from build123d import *

# Parameters (mm, degrees)
SKETCH1_W               = 53
SKETCH1_H               = 53
BOSS_EXTRUDE1_DEPTH     = 1.5
SKETCH2_W               = 16
SKETCH2_H               = 9
CUT_EXTRUDE1_DEPTH      = 75.968326645
SKETCH3_W               = 4.5
SKETCH3_H               = 8
BOSS_EXTRUDE2_DEPTH     = 3
SKETCH4_W               = 1.5
SKETCH4_H               = 5.000000074
CUT_EXTRUDE2_DEPTH      = 3
MIRROR2_COPY_1_SKETCH_W = 4.5
MIRROR2_COPY_1_SKETCH_H = 8
MIRROR2_COPY_1_DEPTH    = 3
MIRROR2_COPY_2_SKETCH_W = 1.5
MIRROR2_COPY_2_SKETCH_H = 5.000000074
MIRROR2_COPY_2_DEPTH    = 3


with BuildPart() as part:
    # Sketch1 → Boss-Extrude1 (new body)
    with BuildSketch(Plane.XY.offset(1.5)):
        with Locations((26.5, 26.5)):
            Rectangle(SKETCH1_W, SKETCH1_H)
    extrude(amount=-BOSS_EXTRUDE1_DEPTH)

    # Sketch2 → Cut-Extrude1 (cut, through all)
    with BuildSketch(Plane(origin=(0, 0, 0), x_dir=(-1, 0, 0), z_dir=(0, 0, -1))):
        with Locations((-26.5, 35.333333333)):
            Rectangle(SKETCH2_W, SKETCH2_H)
    extrude(amount=-CUT_EXTRUDE1_DEPTH, mode=Mode.SUBTRACT)

    # Sketch3 → Boss-Extrude2 (add)
    with BuildSketch(Plane.XY.offset(1.5)):
        with Locations((3.75, 47.5)):
            Rectangle(SKETCH3_W, SKETCH3_H)
    boss_extrude2 = extrude(amount=BOSS_EXTRUDE2_DEPTH)

    # Sketch4 → Cut-Extrude2 (cut)
    with BuildSketch(Plane.XY.offset(4.5)):
        with Locations((3.75, 47.5)):
            Rectangle(SKETCH4_W, SKETCH4_H)
    cut_extrude2 = extrude(amount=-CUT_EXTRUDE2_DEPTH, mode=Mode.SUBTRACT)

    # Mirror1: Boss-Extrude2, Cut-Extrude2 across plane
    add(boss_extrude2.mirror(Plane.ZY.offset(-26.5)))
    add(cut_extrude2.mirror(Plane.ZY.offset(-26.5)), mode=Mode.SUBTRACT)

    # Mirror2: Boss-Extrude2, Cut-Extrude2 across plane
    add(boss_extrude2.mirror(Plane.ZX.offset(26.5)))
    add(cut_extrude2.mirror(Plane.ZX.offset(26.5)), mode=Mode.SUBTRACT)

    # Mirror2 copy 1 sketch → Mirror2 copy 1 (add)
    with BuildSketch(Plane(origin=(53, 53, 1.5), x_dir=(-1, 0, 0), z_dir=(0, 0, 1))):
        with Locations((3.75, 47.5)):
            Rectangle(MIRROR2_COPY_1_SKETCH_W, MIRROR2_COPY_1_SKETCH_H)
    extrude(amount=MIRROR2_COPY_1_DEPTH)

    # Mirror2 copy 2 sketch → Mirror2 copy 2 (cut)
    with BuildSketch(Plane(origin=(53, 53, 4.5), x_dir=(-1, 0, 0), z_dir=(0, 0, 1))):
        with Locations((3.75, 47.5)):
            Rectangle(MIRROR2_COPY_2_SKETCH_W, MIRROR2_COPY_2_SKETCH_H)
    extrude(amount=-MIRROR2_COPY_2_DEPTH, mode=Mode.SUBTRACT)


solid = part.part
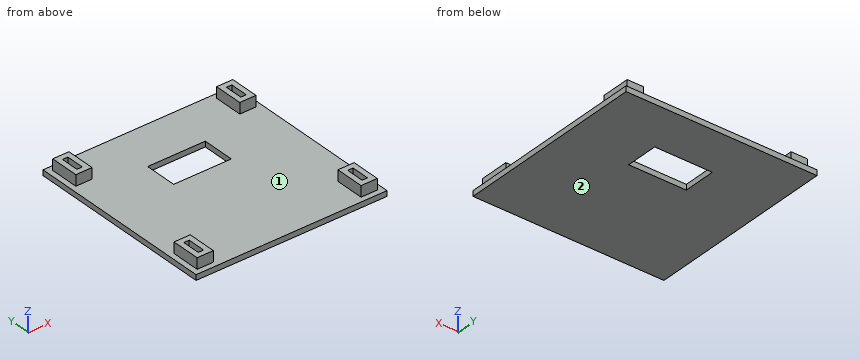
The model under review builds one solid part; all positions refer to its coordinate system, in mm. Face numbers are marked on the shaded views. Round coordinates to 2 decimals unless told otherwise and drop trailing zeros. Write each loop counter-clockwise with the first axis right and the second up, starting at its lowest first coordinate (ties: lowest second). Pieces come first, ordered by that corner, then holes. Notation, with made-up numbers: (-33, -23.5) - (-6, -23.5) arc R22 ccw to (-6, -10.5) - close; hole circle Ø8 at (87, 70.25). An arc over 180 degrees is marked (long way). One line per item, written item: value. Start each with the question number.
1. The part is to be moulded in two halves that separate along X. For the marked faces 1 and 2, say which applies: released by +X, released by -X, zero draft, split by the parting line, or undercut.
2. Consider section C-C on y = 5.5. Write out the cut boundary in (x, z), and give its area (3 significant figures).
3. Consider section B-B on y = 34.5. Write out the cut boundary in (x, z).
4. Consider section A-A on z = 2.15. State how many separate pieces and enclosed holes the cut face has, and give its area (3 significant figures).
5. Consider section D-D on x = 37.5. Write out the cut boundary in (y, z), and give its area (3 significant figures).
6. To check wall thickness, follow L1, parallel to Y at x = 31, z = 1.45; L2, parallel to X at y = 34.5, z = 0.45; L3, parallel to Z at x = 27.5, y = 6.5. State the ranges of each line that lie inside material, in increasing order. Write a range as from..to.
7. Clearance check with flat-ended pins moving along their axes: P1, Ø0.8, axis at x = 4, z = 3, coming from the +Y side; P2, Ø1.5, axis at x = 37, y = 33.5, coming from the -Z side; P3, Ø2.5, axis at y = 6.5, z = 3, coming from the +X side; P4, Ø8, axis at x = 18, y = 12, coming from the +Z side. State where each tip first meets the part, or that it passes through.
Checks:
1. face 1: undercut
1. face 2: zero draft
2. outline: (0, 0) - (53, 0) - (53, 1.5) - (51.5, 1.5) - (51.5, 4.5) - (50, 4.5) - (50, 1.5) - (48.5, 1.5) - (48.5, 4.5) - (47, 4.5) - (47, 1.5) - (6, 1.5) - (6, 4.5) - (4.5, 4.5) - (4.5, 1.5) - (3, 1.5) - (3, 4.5) - (1.5, 4.5) - (1.5, 1.5) - (0, 1.5) - close
2. area: 97.5 mm^2
3. outline: (0, 0) - (18.5, 0) - (18.5, 1.5) - (0, 1.5) - close; (34.5, 0) - (53, 0) - (53, 1.5) - (34.5, 1.5) - close
4. separate pieces: 4
4. enclosed holes: 4
4. area: 114 mm^2
5. outline: (0, 0) - (53, 0) - (53, 1.5) - (0, 1.5) - close
5. area: 79.5 mm^2
6. L1: y = 0..30.83, 39.83..53
6. L2: x = 0..18.5, 34.5..53
6. L3: z = 0..1.5
7. P1: stops at y = 51.5
7. P2: stops at z = 0
7. P3: stops at x = 51.5
7. P4: stops at z = 1.5
